from build123d import *

# Parameters (mm, degrees)
RESSALTO_EXTRUS_O1_DEPTH      = 50
RESSALTO_EXTRUS_O1_DEPTH_BACK = 20
ESBO_O1_R                     = 9.35
ESBO_O1_R_2                   = 7.85
ESBO_O2_R                     = 10.35
ESBO_O2_R_2                   = 9.35
RESSALTO_EXTRUS_O2_DEPTH      = 1
RESSALTO_EXTRUS_O3_START      = -2
ESBO_O3_R                     = 7.85
RESSALTO_EXTRUS_O3_DEPTH      = 2
ESBO_O4_W                     = 12.7
ESBO_O4_H                     = 42
CORTE_EXTRUS_O1_DEPTH         = 21


with BuildPart() as part:
    # Esboço1 → Ressalto-extrusão1 (new, two sides: drawn at the far end of the back side and taken through both)
    with BuildSketch(Plane.XY.offset(-RESSALTO_EXTRUS_O1_DEPTH_BACK)):
        Circle(ESBO_O1_R)
        Circle(ESBO_O1_R_2, mode=Mode.SUBTRACT)
    extrude(amount=RESSALTO_EXTRUS_O1_DEPTH + RESSALTO_EXTRUS_O1_DEPTH_BACK)

    # Esboço2 → Ressalto-extrusão2 (add)
    with BuildSketch(Plane.XY):
        Circle(ESBO_O2_R)
        Circle(ESBO_O2_R_2, mode=Mode.SUBTRACT)
    extrude(amount=RESSALTO_EXTRUS_O2_DEPTH)

    # Esboço3 → Ressalto-extrusão3 (add)
    with BuildSketch(Plane.XY.offset(50).offset(RESSALTO_EXTRUS_O3_START)):
        Circle(ESBO_O3_R)
    extrude(amount=RESSALTO_EXTRUS_O3_DEPTH)

    # Esboço4 → Corte-extrusão1 (cut)
    with BuildSketch(Plane(origin=(0, 0, 0), x_dir=(1, 0, 0), z_dir=(0, 1, 0))):
        with Locations((0, -27)):
            Rectangle(ESBO_O4_W, ESBO_O4_H)
    extrude(amount=CORTE_EXTRUS_O1_DEPTH, mode=Mode.SUBTRACT)


solid = part.part
CAD build for the part. Positions are in the model's coordinates, mm. A direction names the side the tool comes from. Coordinates: 2 decimals unless noted, no trailing zeros. Write each loop counter-clockwise with the first axis right and the second up, starting at its lowest first coordinate (ties: lowest second). Pieces come first, ordered by that corner, then holes. Notation, with made-up numbers: M 27.25,44.25 L 59.25,44.25 A17 ccw 59.25,74.25 Z; hole C 56,52.5 d1. An arc over 180 degrees is marked long. Answer as a JSON object with one key per item and string values. Group by question number.
1) Pin check, flat tips, straight feed: pin 1 Ø2 at (y, z) = (-1, 24) entering from +X; pin 2 Ø1.5 at (x, z) = (1, 13.5) entering from -Y; pin 3 Ø8 at (x, y) = (0.5, -3) entering from -Z. Stop position of each tip, or through.
2) Mould opens along Z. For faces 1 (the face through (-8.21, -6.3, 0.49)), 2 (the face through (-6.35, 6, 27)), 3 (the face through (0, 0, 50)) say: +Z half, -Z half, draft (parallel to the pull), parting line (faces both ways), or undercut.
3) Saw through at C-C (y = 0). Write the cut outline in (x, z).
4) Tool access for faces 4 (the face through (-4.6, -8.4, 1)), 5 (the face through (-1, 8, 6)), 6 (the face through (-4.6, -8.4, 0)), 7 (the face through (-2, 8, -20)): list every direction of +Z, -Z, +X, -X, +Y, -Y with a clear straight run to the whole face (end or side of a thin tool).
5) Wall check: line 1 (Y direction, x = 0, z = -1); line 2 (Z direction, x = 5.75, y = 8.5); line 3 (Z direction, x = 1.75, y = -3.25). Give the ranges that are in metal, low to high. Write a range as from..to.
6) Saw through at B-B (y = 8.5). Write the cut outline in (x, z).
7) Saw through at A-A (x = 0). Write the cut outline in (y, z), plus the area to 3 significant figures.
8) Saw through at D-D (x = 3.25). Write the cut outline in (y, z).
Values follow:
{
 "1": {"pin 1": "stops at x = 9.35", "pin 2": "stops at y = -9.35", "pin 3": "stops at z = 48"},
 "2": {"face 1": "draft", "face 2": "undercut", "face 3": "+Z half"},
 "3": {"outline": "M -10.35,0 L -9.35,0 L -9.35,-20 L -7.85,-20 L -7.85,48 L 7.85,48 L 7.85,-20 L 9.35,-20 L 9.35,0 L 10.35,0 L 10.35,1 L 9.35,1 L 9.35,50 L -9.35,50 L -9.35,1 L -10.35,1 Z"},
 "4": {"face 4": "+Z", "face 5": "+Y", "face 6": "-Z", "face 7": "-Z, +X, -X, +Y, -Y"},
 "5": {"line 1": "y = -9.35..-7.85, 7.85..9.35", "line 2": "z = 0..1", "line 3": "z = 48..50"},
 "6": {"outline": "M -5.91,0 L -3.9,0 L -3.9,-20 L 3.9,-20 L 3.9,0 L 5.91,0 L 5.91,1 L 3.9,1 L 3.9,6 L -3.9,6 L -3.9,1 L -5.91,1 Z; M -3.9,48 L 3.9,48 L 3.9,50 L -3.9,50 Z"},
 "7": {"outline": "M -10.35,0 L -9.35,0 L -9.35,-20 L -7.85,-20 L -7.85,48 L 9.35,48 L 9.35,50 L -9.35,50 L -9.35,1 L -10.35,1 Z; M 7.85,-20 L 9.35,-20 L 9.35,0 L 10.35,0 L 10.35,1 L 9.35,1 L 9.35,6 L 7.85,6 Z", "area": "180 mm2"},
 "8": {"outline": "M -9.83,0 L -8.77,0 L -8.77,-20 L -7.15,-20 L -7.15,48 L 8.77,48 L 8.77,50 L -8.77,50 L -8.77,1 L -9.83,1 Z; M 7.15,-20 L 8.77,-20 L 8.77,0 L 9.83,0 L 9.83,1 L 8.77,1 L 8.77,6 L 7.15,6 Z"}
}
